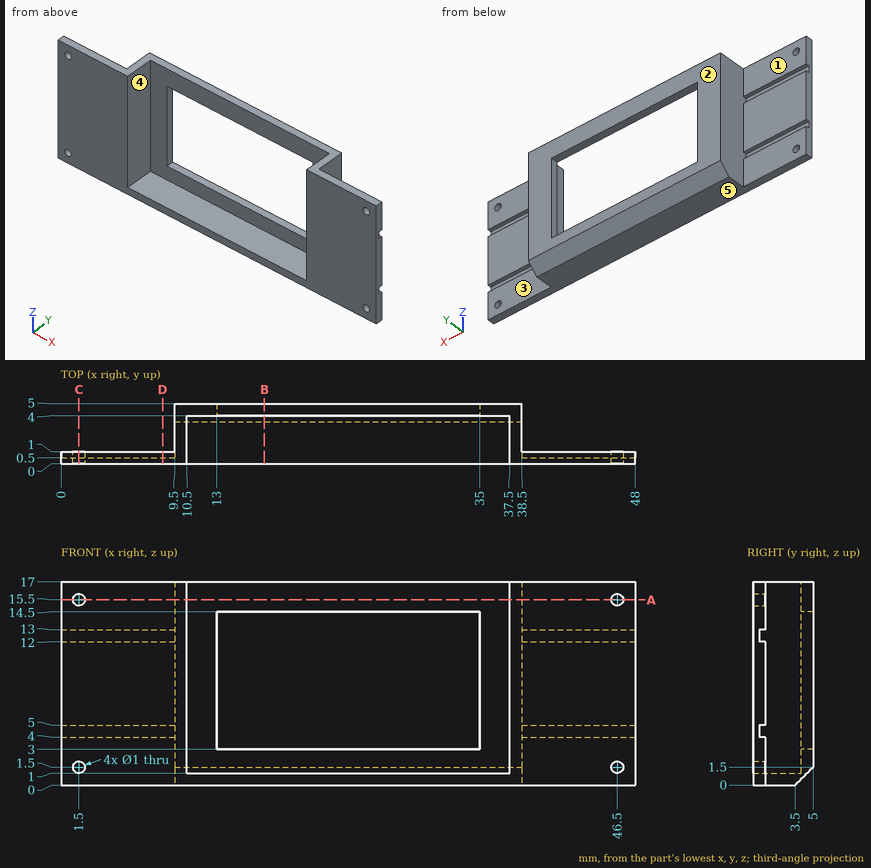
Verification items for this drawing (mm, ordinates from the low corner). A direction names the side the tool comes from. Coordinates: 2 decimals unless noted, no trailing zeros. Write each loop counter-clockwise with the first axis right and the second up, starting at its lowest first coordinate (ties: lowest second). Pieces come first, ordered by that corner, then holes. Notation, with made-up numbers: (-21.5, 36.25) -> (30.5, 36.25) arc R12 cw to (30.5, 40.25) -> close; hole circle Ø5 at (78.25, 50). An arc over 180 degrees is marked (long way). One line per item, written item: value. Start each with the question number.
Q1. Cross-section at A-A on z = 15.5. Enter the section's corners in (x, y), and give its area (3 significant figures).
Q2. Thickness scan on L1, parallel to Z at x = 1.5, y = 0.55; L2, parallel to Z at x = 46.5, y = 0.4; L3, parallel to X at y = 2.45, z = 1.25. Record the ranges inside material, lowest first. Write a range as from..to.
Q3. Cross-section at B-B on x = 17. Enter the section's corners in (y, z).
Q4. Cross-section at C-C on x = 1.5. Enter the section's corners in (y, z).
Q5. Access from +Z, -Z, +X, -X, +Y, -Y to the whole of each face (thin tool, end or side, straight path). Record for the marked faces 1, 2, 3, 4 and 5.
Q6. Cross-section at D-D on x = 8.5. Enter the section's corners in (y, z), and give its area (3 significant figures).
Q7. Go/stop test with flat-tipped pins: P1, Ø1.5, axis at x = 40.5, z = 7, coming from the +Y side; P2, Ø0.5, axis at x = 43.5, z = 12.5, coming from the +Y side; P3, Ø1, axis at y = 3.5, z = 15, coming from the +X side. Record where each tip stops, or that it passes through.
Checked values:
1. outline: (0, 0) -> (1, 0) -> (1, 1) -> (0, 1) -> close; (2, 0) -> (10.5, 0) -> (10.5, 4) -> (37.5, 4) -> (37.5, 0) -> (46, 0) -> (46, 1) -> (38.5, 1) -> (38.5, 5) -> (9.5, 5) -> (9.5, 1) -> (2, 1) -> close; (47, 0) -> (48, 0) -> (48, 1) -> (47, 1) -> close
1. area: 54.0 mm²
2. L1: z = 0..1, 2..4, 5..12, 13..15, 16..17
2. L2: z = 0..1, 2..15, 16..17
2. L3: x = 9.5..10.5, 37.5..38.5
3. outline: (0, 0) -> (3.5, 0) -> (5, 1.5) -> (5, 3) -> (4, 3) -> (4, 1) -> (0, 1) -> close; (4, 14.5) -> (5, 14.5) -> (5, 17) -> (4, 17) -> close
4. outline: (0, 0) -> (1, 0) -> (1, 1) -> (0, 1) -> close; (0, 2) -> (1, 2) -> (1, 4) -> (0.5, 4) -> (0.5, 5) -> (1, 5) -> (1, 12) -> (0.5, 12) -> (0.5, 13) -> (1, 13) -> (1, 15) -> (0, 15) -> close; (0, 16) -> (1, 16) -> (1, 17) -> (0, 17) -> close
5. face 1: +Z, -Z, -X, +Y
5. face 2: +Z, -Z, +X, -X, +Y
5. face 3: +Z, -Z, +X, +Y
5. face 4: +Z, -Y
5. face 5: -Z, +X, -X, +Y, -Y
6. outline: (0, 0) -> (1, 0) -> (1, 4) -> (0.5, 4) -> (0.5, 5) -> (1, 5) -> (1, 12) -> (0.5, 12) -> (0.5, 13) -> (1, 13) -> (1, 17) -> (0, 17) -> close
6. area: 16.0 mm²
7. P1: stops at y = 1
7. P2: stops at y = 0.5
7. P3: stops at x = 38.5
